Here's how the part is built. I have some questions about the finished solid (model axes, mm). A direction names the side the tool comes from. Coordinates: 2 decimals unless noted, no trailing zeros. Write each loop counter-clockwise with the first axis right and the second up, starting at its lowest first coordinate (ties: lowest second). Pieces come first, ordered by that corner, then holes. Notation, with made-up numbers: M 47,13 L 58,13 A14 ccw 58,22 Z; hole C -16.75,78 d9. An arc over 180 degrees is marked long. Use one line per item in the form item = value. Start each with the question number.
1. Thinking about a two-plate mould opening in X: for faces 1 (the face through (25, 8, 94)), 2 (the face through (40, 8, 20)), 3 (the face through (0, 7, 46)), which applies, released by +X, released by -X, zero draft, split by the parting line, or undercut?
2. Please list where these lines run through material, in increasing order: line 1 along Y through (x, z) = (40, 5); line 2 along X through (y, z) = (5.75, 14.5); line 3 along X through (y, z) = (9, 84). Write a range as [from, to].
3. I want a section at D-D, the plane x = 40. List the corners of the cut face in (y, z) for me.
4. On a 3-axis mill with a long thin cutter (end or side, diameter ignored), from which of +Z, -Z, +X, -X, +Y, -Y can I reach the whole of each face in a straight line? I mean faces 4 (the face through (40, 8, 74)), 5 (the face through (25, 15, 36)), 6 (the face through (37.69, 6.54, 10.37)). Say none if no direction works.
5. I want a section at A-A, the plane x = 25. List the corners of the cut face in (y, z) for me, plus the area to 3 significant figures.
6. I want a section at C-C, the plane z = 46. List the corners of the cut face in (x, y) for me.
7. I'm going to push flat-ended pins straight in: pin 1 Ø2.5 at (x, y) = (11, 8) entering from +Z; pin 2 Ø3 at (x, y) = (40, 7.5) entering from -Z; pin 3 Ø4 at (x, y) = (9, 7) entering from -Z. Where does each tip first touch, or does it pass through?
from build123d import *

# Parameters (mm, degrees)
SZKIC1_W                    = 50
SZKIC1_H                    = 15
DODANIE_WYCI_GNI_CIE1_DEPTH = 47
SZKIC2_R                    = 2.5
WYTNIJ_WYCI_GNI_CIE1_DEPTH  = 20
LUSTRO1_START               = 47
LUSTRO1_OUTLINE_W           = 50
LUSTRO1_OUTLINE_H           = 15
LUSTRO1_OUTLINE_R           = 2.5
LUSTRO1_DEPTH               = 47
LUSTRO1_2_OUTLINE_R         = 2.5
LUSTRO1_2_DEPTH             = 27
SZKIC5_R                    = 7
WYTNIJ_WYCI_GNI_CIE2_DEPTH  = 108.522090753
SFAZOWANIE2_SIZE            = 1


# Read off the part's stored shape, not the designer's step: Lustro1
with BuildPart() as part:
    # Szkic1 → Dodanie-wyciągnięcie1 (new body)
    with BuildSketch(Plane.XY):
        with Locations((25, 7.5)):
            Rectangle(SZKIC1_W, SZKIC1_H)
    extrude(amount=DODANIE_WYCI_GNI_CIE1_DEPTH)

    # Szkic2 → Wytnij-wyciągnięcie1 (cut)
    with BuildSketch(Plane(origin=(0, 0, 0), x_dir=(-1, 0, 0), z_dir=(0, 0, -1))):
        with Locations((-40, 7.5)):
            Circle(SZKIC2_R)
        with Locations((-10, 7.5)):
            Circle(SZKIC2_R)
    extrude(amount=-WYTNIJ_WYCI_GNI_CIE1_DEPTH, mode=Mode.SUBTRACT)

    # Lustro1 outline → Lustro1 (add)
    with BuildSketch(Plane.XY.offset(LUSTRO1_START)):
        with Locations((25, 7.5)):
            Rectangle(LUSTRO1_OUTLINE_W, LUSTRO1_OUTLINE_H)
        with Locations((10, 7.5)):
            Circle(LUSTRO1_OUTLINE_R, mode=Mode.SUBTRACT)
        with Locations((40, 7.5)):
            Circle(LUSTRO1_OUTLINE_R, mode=Mode.SUBTRACT)
    extrude(amount=LUSTRO1_DEPTH)

    # Lustro1 2 outline → Lustro1 2 (add)
    with BuildSketch(Plane.XY.offset(LUSTRO1_START)):
        with Locations((10, 7.5)):
            Circle(LUSTRO1_2_OUTLINE_R)
        with Locations((40, 7.5)):
            Circle(LUSTRO1_2_OUTLINE_R)
    extrude(amount=LUSTRO1_2_DEPTH)

    # Szkic5 → Wytnij-wyciągnięcie2 (cut, through all)
    with BuildSketch(Plane(origin=(0, 15, 0), x_dir=(1, 0, 0), z_dir=(0, 1, 0))):
        with Locations(Location((25, -47, 0), (0, 0, 270))):
            Circle(SZKIC5_R)
    extrude(amount=-WYTNIJ_WYCI_GNI_CIE2_DEPTH, mode=Mode.SUBTRACT)

    # Sfazowanie2
    sfazowanie2_edges = [part.edges().sort_by_distance(p)[0] for p in [
        (42.5, 7.5, 0),
        (12.5, 7.5, 0),
        (37.5, 7.5, 94),
        (7.5, 7.5, 94),
    ]]
    chamfer(sfazowanie2_edges, length=SFAZOWANIE2_SIZE)


solid = part.part
Answer list:
q1.face_1 = zero draft
q1.face_2 = undercut
q1.face_3 = released by -X
q2.line_1 = [0, 5], [10, 15]
q2.line_2 = [0, 8.21], [11.79, 38.21], [41.79, 50]
q2.line_3 = [0, 8], [12, 38], [42, 50]
q3.outline = M 0,0 L 4,0 L 5,1 L 5,20 L 10,20 L 10,1 L 11,0 L 15,0 L 15,94 L 11,94 L 10,93 L 10,74 L 5,74 L 5,93 L 4,94 L 0,94 Z
q4.face_4 = +Z
q4.face_5 = +Z, -Z, +X, -X, +Y
q4.face_6 = -Z
q5.outline = M 0,0 L 15,0 L 15,40 L 0,40 Z; M 0,54 L 15,54 L 15,94 L 0,94 Z
q5.area = 1,200 mm²
q6.outline = M 0,0 L 18.07,0 L 18.07,15 L 0,15 Z; M 31.93,0 L 50,0 L 50,15 L 31.93,15 Z
q7.pin_1 = 74
q7.pin_2 = 20
q7.pin_3 = 0.38
